Job drawing, mm, ordinate dimensions from the low corner. One solid piece. A direction names the side the tool comes from. Coordinates: 2 decimals unless noted, no trailing zeros. Order: outer loops, then holes, each group sorted by start corner. A loop starts at its lowest first (then second) coordinate and runs counter-clockwise, first axis right, second up. Notation, with made-up numbers: (47.25, -37) - (90.25, -37) arc R26 ccw to (90.25, -5) - close; hole circle Ø8 at (60, -7.75). An arc over 180 degrees is marked (long way). Use a Markdown table: item, result. Add a question column.
1) Saw through at D-D on z = 9. List the corners of the cut face in (x, y), then the cut area to 3 significant figures.
2) Two-plate mould, pull along X, no slides. Class the marked faces 1, 2, 3 and 4: +X half, -X half, draft (parallel to the pull), parting line (faces both ways), or undercut.
3) Saw through at B-B on x = 35. List the corners of the cut face in (y, z), then the cut area to 4 significant figures.
4) Wall check: L1, parallel to X at y = 13.5, z = 34; L2, parallel to X at y = 3.85, z = 35; L3, parallel to Z at x = 61, y = 10.25. Give the ranges that are in metal, low to high. Write a range as [from, to].
5) Tool access for the marked faces 5 and 6: list every direction of +Z, -Z, +X, -X, +Y, -Y with a clear straight run to the whole face (end or side of a thin tool).
6) Drop flat-ended pins along their axis: P1, Ø5, axis at x = 47.5, y = 7.5, coming from the -Z side; P2, Ø2, axis at x = 55.5, y = 12, coming from the -Z side; P3, Ø6, axis at y = 10.5, z = 19, coming from the +X side. Give the stop position or say it passes through.
7) Saw through at C-C on x = 20. List the corners of the cut face in (y, z), then the cut area to 3 significant figures.
8) Saw through at A-A on z = 35. List the corners of the cut face in (x, y).
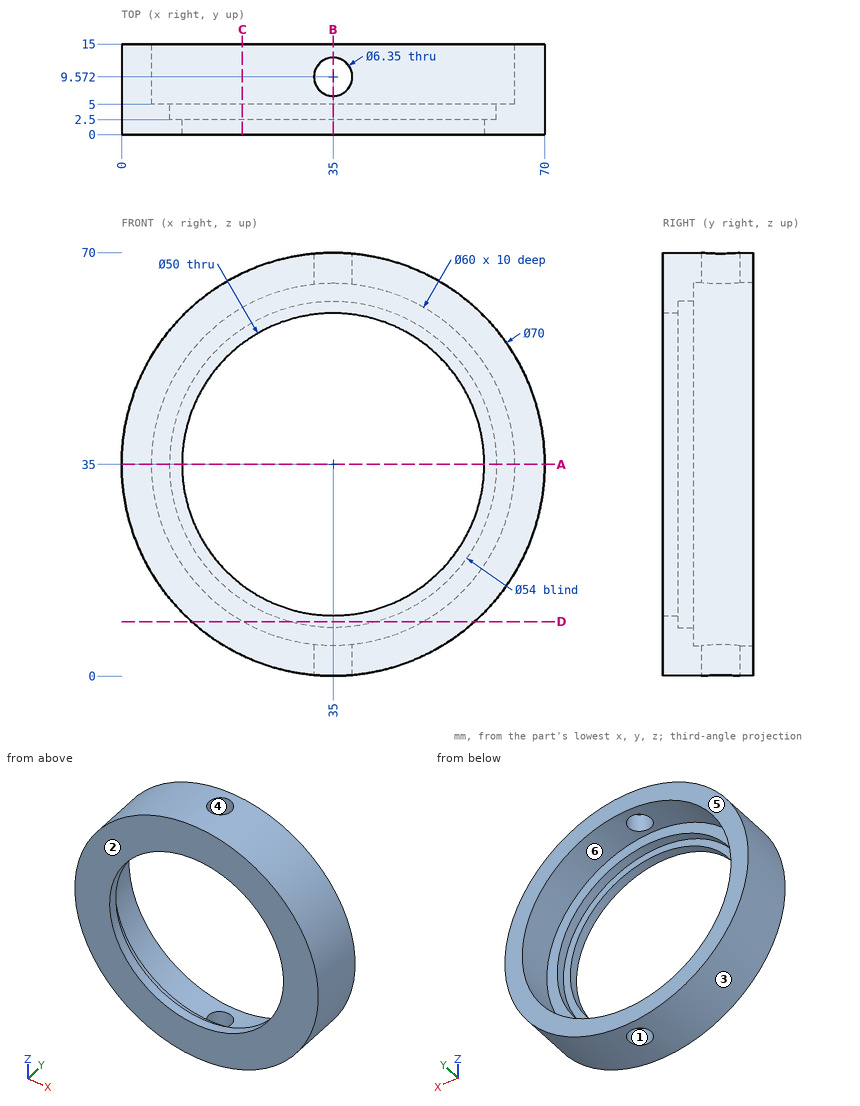
Results are:
| question | item | result |
|---|---|---|
| 1 | outline | (11.57, 0) - (58.43, 0) - (58.43, 15) - (49.97, 15) - (49.97, 5) - (42.28, 5) - (42.28, 2.5) - (27.72, 2.5) - (27.72, 5) - (20.03, 5) - (20.03, 15) - (11.57, 15) - close |
| 1 | area | 367 mm2 |
| 2 | face 1 | undercut |
| 2 | face 2 | draft |
| 2 | face 3 | parting line |
| 2 | face 4 | undercut |
| 3 | outline | (0, 0) - (6.4, 0) - (6.4, 5) - (5, 5) - (5, 8) - (2.5, 8) - (2.5, 10) - (0, 10) - close; (0, 60) - (2.5, 60) - (2.5, 62) - (5, 62) - (5, 65) - (6.4, 65) - (6.4, 70) - (0, 70) - close; (12.75, 0) - (15, 0) - (15, 5) - (12.75, 5) - close; (12.75, 65) - (15, 65) - (15, 70) - (12.75, 70) - close |
| 3 | area | 126.5 mm2 |
| 4 | L1 | [0.01, 5.02], [64.98, 69.99] |
| 4 | L2 | [0, 8], [62, 70] |
| 4 | L3 | [11.57, 20.03], [49.97, 58.43] |
| 5 | face 5 | +Z, -Z, +X, -X, +Y |
| 5 | face 6 | +Y |
| 6 | P1 | z = 1.46 |
| 6 | P2 | z = 5.94 |
| 6 | P3 | x = 67.5 |
| 7 | outline | (0, 3.38) - (15, 3.38) - (15, 9.02) - (5, 9.02) - (5, 12.55) - (2.5, 12.55) - (2.5, 15) - (0, 15) - close; (0, 55) - (2.5, 55) - (2.5, 57.45) - (5, 57.45) - (5, 60.98) - (15, 60.98) - (15, 66.62) - (0, 66.62) - close |
| 7 | area | 217 mm2 |
| 8 | outline | (0, 0) - (10, 0) - (10, 2.5) - (8, 2.5) - (8, 5) - (5, 5) - (5, 15) - (0, 15) - close; (60, 0) - (70, 0) - (70, 15) - (65, 15) - (65, 5) - (62, 5) - (62, 2.5) - (60, 2.5) - close |
